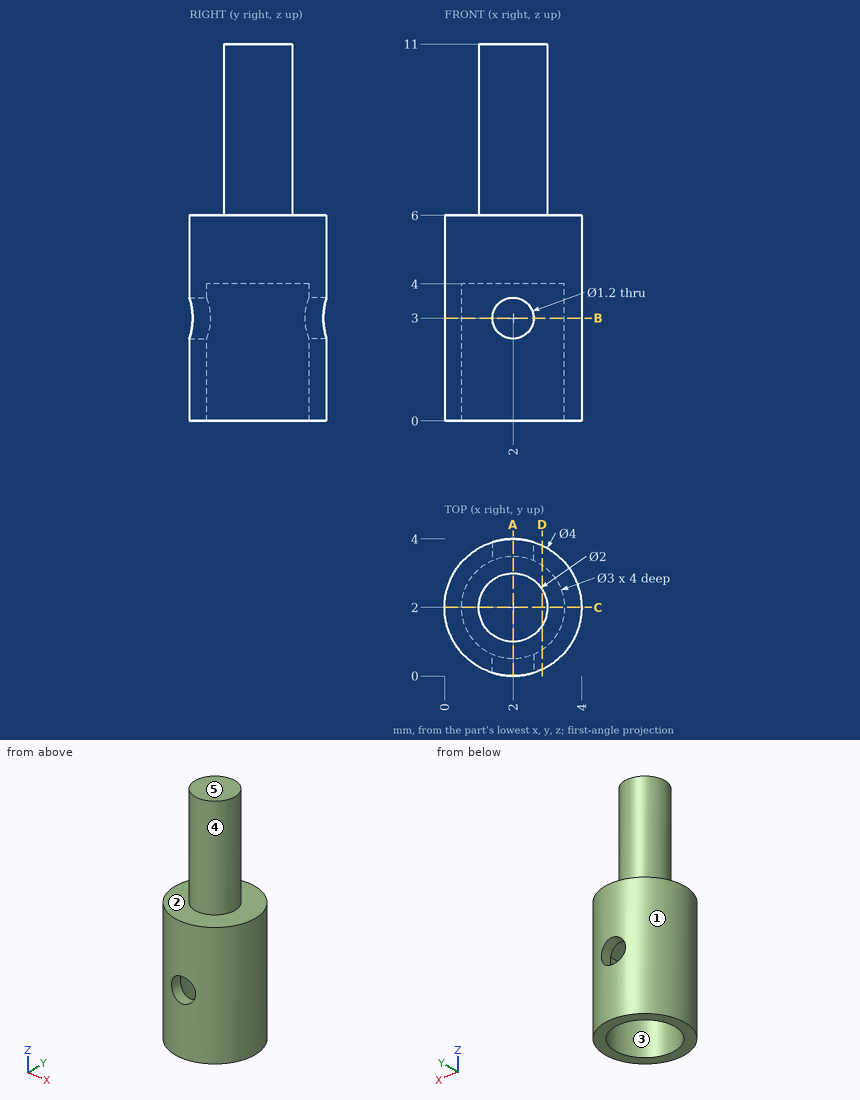
Job drawing, mm, ordinate dimensions from the low corner. One solid piece. A direction names the side the tool comes from. Round coordinates to 2 decimals unless told otherwise and drop trailing zeros. Loops run counter-clockwise (first coordinate to the right, second up) from the corner with the lowest first, then second, coordinate; pieces in that order, holes last. Notation, with made-up numbers: M -2,-21 L 10,-21 A30 cw 10,13 Z; hole C -36.5,72.5 d8. An arc over 180 degrees is marked long. One line per question, with ' | ' between items. Start each with the question number.
Item 1: Cut at B-B, the plane z = 3. Write the cut outline in (x, y).
Item 2: Wall check: line 1 (Z direction, x = 0.8, y = 3.45); line 2 (Y direction, x = 2.9, z = 2.5); line 3 (Z direction, x = 1.6, y = 3.35). Give the ranges that are in metal, low to high.
Item 3: Which spindle directions (+Z, -Z, +X, -X, +Y, -Y) get a long thin tool onto all of the face, cutting with end or side? Do the marked faces 1 and 2. Say none if no direction does.
Item 4: Pin check, flat tips, straight feed: pin 1 Ø1.5 at (x, y) = (2.5, 2) entering from -Z; pin 2 Ø1.5 at (y, z) = (1, 4.5) entering from +X. Stop position of each tip, or through.
Item 5: Cut at C-C, the plane y = 2. Write the cut outline in (x, z).
Item 6: Cut at D-D, the plane x = 2.85. Write the cut outline in (y, z).
Item 7: Cut at A-A, the plane x = 2. Write the cut outline in (y, z), plus the area to 3 significant figures.
Item 8: Two-plate mould, pull along X, no slides. Class the marked faces 3, 4 and 5: pulls with the +X half, pulls with the -X half, needs draft (parallel to the pull), parting line crosses it, or undercut.
Responses:
1) outline: M 1.4,0.09 L 1.4,0.63 A1.5 cw 1.4,3.37 L 1.4,3.91 A2 ccw Z; M 2.6,0.09 A2 ccw 2.6,3.91 L 2.6,3.37 A1.5 cw 2.6,0.63 Z
2) line 1: z = 0 to 6 | line 2: y = 0.21 to 0.8, 3.2 to 3.79 | line 3: z = 4 to 6
3) face 1: +Z, -Z | face 2: +Z
4) pin 1: stops at z = 4 | pin 2: stops at x = 3.98
5) outline: M 0,0 L 0.5,0 L 0.5,4 L 3.5,4 L 3.5,0 L 4,0 L 4,6 L 3,6 L 3,11 L 1,11 L 1,6 L 0,6 Z
6) outline: M 0.19,0 L 0.76,0 L 0.76,4 L 3.24,4 L 3.24,0 L 3.81,0 L 3.81,6 L 2.53,6 L 2.53,11 L 1.47,11 L 1.47,6 L 0.19,6 Z
7) outline: M 0,0 L 0.5,0 L 0.5,2.4 L 0,2.4 Z; M 0,3.6 L 0.5,3.6 L 0.5,4 L 3.5,4 L 3.5,3.6 L 4,3.6 L 4,6 L 3,6 L 3,11 L 1,11 L 1,6 L 0,6 Z; M 3.5,0 L 4,0 L 4,2.4 L 3.5,2.4 Z | area: 20.8 mm²
8) face 3: undercut | face 4: parting line crosses it | face 5: needs draft
